Design review of the part built by this model. Coordinates are the model's own, in mm. Face numbers are marked on the shaded views. A direction names the side the tool comes from. Give positions to 0.01 mm unless a question says otherwise; leave off trailing zeros. Order: outer loops, then holes, each group sorted by start corner. A loop starts at its lowest first (then second) coordinate and runs counter-clockwise, first axis right, second up.
```python
from build123d import *

# Parameters (mm, degrees)
F1_DEPTH = 8
F2_T     = -1
F4_DEPTH = 1


with BuildPart() as f1:
    # F0 (on Top) → F1 (new body)
    with BuildSketch(Plane.XY):
        with BuildLine():
            Line((-13.65, -7.45), (13.65, -7.45))
            ThreePointArc((13.65, -7.45), (15.7713203436, -6.5713203436), (16.65, -4.45))
            Line((16.65, -4.45), (16.65, 4.45))
            ThreePointArc((16.65, 4.45), (15.7713203436, 6.5713203436), (13.65, 7.45))
            Line((13.65, 7.45), (-13.65, 7.45))
            ThreePointArc((-13.65, 7.45), (-15.7713203436, 6.5713203436), (-16.65, 4.45))
            Line((-16.65, 4.45), (-16.65, -4.45))
            ThreePointArc((-16.65, -4.45), (-15.7713203436, -6.5713203436), (-13.65, -7.45))
        make_face()
    extrude(amount=F1_DEPTH)

    # F2
    f2_openings = [f1.faces().sort_by_distance(p)[0] for p in [
        (0, 0, 8),
    ]]
    offset(amount=F2_T, openings=f2_openings)

    # F3 (on face) → F4 (join)
    with BuildSketch(Plane(origin=(0, 0, 0), x_dir=(1, 0, 0), z_dir=(0, 0, -1))):
        with BuildLine():
            Line((-14.5, -8.25), (14.5, -8.25))
            ThreePointArc((14.5, -8.25), (16.6213203436, -7.3713203436), (17.5, -5.25))
            Line((17.5, -5.25), (17.5, 5.25))
            ThreePointArc((17.5, 5.25), (16.6213203436, 7.3713203436), (14.5, 8.25))
            Line((14.5, 8.25), (-14.5, 8.25))
            ThreePointArc((-14.5, 8.25), (-16.6213203436, 7.3713203436), (-17.5, 5.25))
            Line((-17.5, 5.25), (-17.5, -5.25))
            ThreePointArc((-17.5, -5.25), (-16.6213203436, -7.3713203436), (-14.5, -8.25))
        make_face()
        with BuildLine():
            Line((-13.65, 7.45), (13.65, 7.45))
            ThreePointArc((13.65, 7.45), (15.7713203436, 6.5713203436), (16.65, 4.45))
            Line((16.65, 4.45), (16.65, -4.45))
            ThreePointArc((16.65, -4.45), (15.7713203436, -6.5713203436), (13.65, -7.45))
            Line((13.65, -7.45), (-13.65, -7.45))
            ThreePointArc((-13.65, -7.45), (-15.7713203436, -6.5713203436), (-16.65, -4.45))
            Line((-16.65, -4.45), (-16.65, 4.45))
            ThreePointArc((-16.65, 4.45), (-15.7713203436, 6.5713203436), (-13.65, 7.45))
        make_face(mode=Mode.SUBTRACT)
    extrude(amount=-F4_DEPTH)


solid = f1.part
```
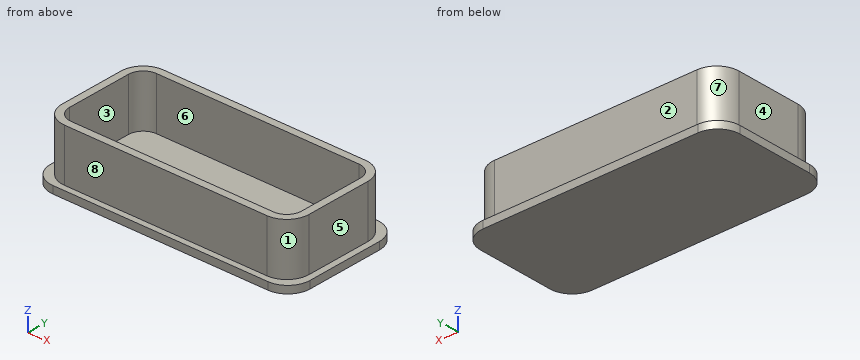
1. Take a section at C-C (y = -1.25). State the section outline as (x, z) points.
Recorded:
outline: (-17.5, 0) - (17.5, 0) - (17.5, 1) - (16.65, 1) - (16.65, 8) - (15.65, 8) - (15.65, 1) - (-15.65, 1) - (-15.65, 8) - (-16.65, 8) - (-16.65, 1) - (-17.5, 1) - close
2. For pin 1 (1.5 mm diameter, centred on y = -3, z = 4, fed in from -X); pin 2 (1 mm diameter, centred on x = 14, z = 6.5, fed in from -Y); pin 3 (2 mm diameter, centred on x = -5.5, z = 3, fed in from +Y), all flat-tipped, find the tip position at first contact; note any pin that passes through.
Recorded:
pin 1: stops at x = -16.65
pin 2: stops at y = -7.45
pin 3: stops at y = 7.45
3. Draft analysis for pull direction X (two halves, no side actions). For the marked faces 1, 2 and 3, state which applies: pulls with the +X half, pulls with the -X half, needs draft (parallel to the pull), parting line crosses it, or undercut.
Recorded:
face 1: pulls with the +X half
face 2: needs draft
face 3: undercut
4. Machinability: for the marked faces 4, 5, 6, 7 and 8, which of the approach directions +Z, -Z, +X, -X, +Y, -Y give a long, thin tool a straight path to every point of the face, cutting with its end or side? Answer none if there is none.
Recorded:
face 4: +Z, -X, +Y, -Y
face 5: +Z, +X, +Y, -Y
face 6: +Z
face 7: +Z, -X, +Y
face 8: +Z, +X, -X, -Y
5. Take a section at B-B (x = -11). State the section outline as (y, z) points.
Recorded:
outline: (-8.25, 0) - (8.25, 0) - (8.25, 1) - (7.45, 1) - (7.45, 8) - (6.45, 8) - (6.45, 1) - (-6.45, 1) - (-6.45, 8) - (-7.45, 8) - (-7.45, 1) - (-8.25, 1) - close
6. For line 1 along Y through (x, z) = (-10, 7); line 2 along X through (y, z) = (2, 4.5); line 3 along Z through (x, y) = (-11.5, -5.25), list the stretches that pass through material, from the lowest coordinate up.
Recorded:
line 1: y = -7.45 to -6.45, 6.45 to 7.45
line 2: x = -16.65 to -15.65, 15.65 to 16.65
line 3: z = 0 to 1
7. Take a section at A-A (z = 1.5). State the section outline as (x, y) points, then the cut area to 3 significant figures.
Recorded:
outline: (-16.65, -4.45) arc R3 ccw to (-13.65, -7.45) - (13.65, -7.45) arc R3 ccw to (16.65, -4.45) - (16.65, 4.45) arc R3 ccw to (13.65, 7.45) - (-13.65, 7.45) arc R3 ccw to (-16.65, 4.45) - close; hole (-15.65, -4.45) arc R2 ccw to (-13.65, -6.45) - (13.65, -6.45) arc R2 ccw to (15.65, -4.45) - (15.65, 4.45) arc R2 ccw to (13.65, 6.45) - (-13.65, 6.45) arc R2 ccw to (-15.65, 4.45) - close
area: 88.1 mm2
